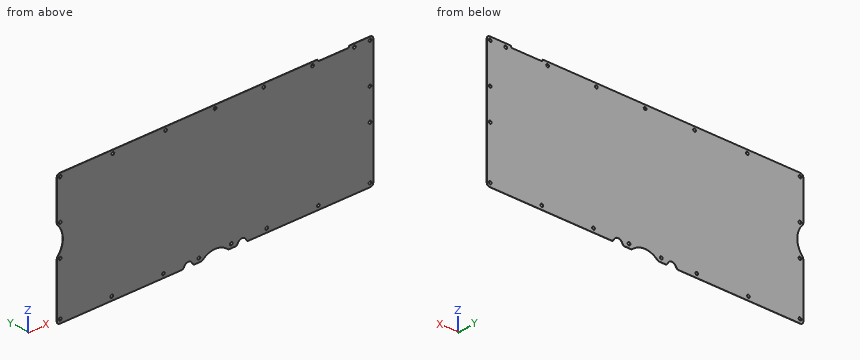
from build123d import *

# Parameters (mm, degrees)
SKETCH1_W                 = 373.38
SKETCH1_H                 = 149.225
BOSS_EXTRUDE1_DEPTH       = 0.254
F_4_CLEARANCE_HOLE2_D     = 3.2639
F_4_CLEARANCE_HOLE2_DEPTH = 0.762
F_4_CLEARANCE_HOLE2_TIP   = 0.980574487
CUT_EXTRUDE2_REACH        = 203.048
SKETCH7_R                 = 22.225
FILLET2_R                 = 3.175
F_4_CLEARANCE_HOLE3_D     = 3.2639
SKETCH10_R                = 5.334
CUT_EXTRUDE3_DEPTH        = 1.016
FILLET3_R                 = 3.175
SKETCH11_R                = 22.86
CUT_EXTRUDE4_DEPTH        = 202.047869355
FILLET4_R                 = 3.175
F_4_CLEARANCE_HOLE4_D     = 3.2639
SKETCH15_W                = 36.703
SKETCH15_H                = 2.6035
CUT_EXTRUDE5_DEPTH        = 202.047869355
F_4_CLEARANCE_HOLE5_D     = 3.2639
SKETCH20_W                = 373.38
SKETCH20_H                = 0.635
CUT_EXTRUDE6_DEPTH        = 202.047869355
FILLET6_R                 = 0.762
FILLET7_R                 = 3.175


with BuildPart() as part:
    # Sketch1 → Boss-Extrude1 (new body)
    with BuildSketch(Plane(origin=(0, 0, 0), x_dir=(1, 0, 0), z_dir=(0, 1, 0))):
        Rectangle(SKETCH1_W, SKETCH1_H)
    extrude(amount=BOSS_EXTRUDE1_DEPTH)

    # #4 Clearance Hole2
    with Locations(Plane(origin=(0, 0.254, 0), x_dir=(-1, 0, 0), z_dir=(0, 1, 0))):
        with Locations((121.92, -70.1675), (60.96, -70.1675), (0, -70.1675), (-60.96, -70.1675), (-121.92, -70.1675)):
            Hole(F_4_CLEARANCE_HOLE2_D / 2, depth=F_4_CLEARANCE_HOLE2_DEPTH)
            with Locations((0, 0, -(F_4_CLEARANCE_HOLE2_DEPTH + F_4_CLEARANCE_HOLE2_TIP / 2))):  # 118° drill point
                Cone(0, F_4_CLEARANCE_HOLE2_D / 2, F_4_CLEARANCE_HOLE2_TIP, mode=Mode.SUBTRACT)

    # Sketch7 → Cut-Extrude2 (cut, up to next)
    with BuildSketch(Plane(origin=(0, 0.254, 0), x_dir=(1, 0, 0), z_dir=(0, 1, 0)), mode=Mode.PRIVATE) as cut_extrude2_sk1:
        with Locations((0, 90.4875)):
            Circle(SKETCH7_R)
    cut_extrude2_tool1 = extrude(cut_extrude2_sk1.sketch, amount=-CUT_EXTRUDE2_REACH, mode=Mode.PRIVATE) & part.part
    add(cut_extrude2_tool1.solids().sort_by_distance((0, 0.254, -90.4875))[0], mode=Mode.SUBTRACT)

    # Fillet2
    fillet2_edges = [part.edges().sort_by_distance(p)[0] for p in [
        (15.554259867, 0.127, -74.6125),
        (-15.554259867, 0.127, -74.6125),
    ]]
    fillet(fillet2_edges, radius=FILLET2_R)

    # #4 Clearance Hole3 (through all)
    with Locations(Plane(origin=(0, 0.254, 0), x_dir=(-1, 0, 0), z_dir=(0, 1, 0))):
        with Locations((19.05, -70.1675), (-19.05, -70.1675)):
            Hole(F_4_CLEARANCE_HOLE3_D / 2)

    # Sketch10 → Cut-Extrude3 (cut)
    with BuildSketch(Plane(origin=(0, 0.254, 0), x_dir=(1, 0, 0), z_dir=(0, 1, 0))):
        with Locations((31.75, 74.6125)):
            Circle(SKETCH10_R)
        with Locations((-31.75, 74.6125)):
            Circle(SKETCH10_R)
    extrude(amount=-CUT_EXTRUDE3_DEPTH, mode=Mode.SUBTRACT)

    # Fillet3
    fillet3_edges = [part.edges().sort_by_distance(p)[0] for p in [
        (37.084, 0.127, -74.6125),
        (26.416, 0.127, -74.6125),
        (-26.416, 0.127, -74.6125),
        (-37.084, 0.127, -74.6125),
    ]]
    fillet(fillet3_edges, radius=FILLET3_R)

    # Sketch11 → Cut-Extrude4 (cut, through all)
    with BuildSketch(Plane(origin=(0, 0.254, 0), x_dir=(1, 0, 0), z_dir=(0, 1, 0))):
        with Locations((-202.565, -7.9375)):
            Circle(SKETCH11_R)
    extrude(amount=-CUT_EXTRUDE4_DEPTH, mode=Mode.SUBTRACT)

    # Fillet4
    fillet4_edges = [part.edges().sort_by_distance(p)[0] for p in [
        (-186.69, 0.127, -8.511328986),
        (-186.69, 0.127, 24.386328986),
        (-186.69, 0.127, -74.6125),
        (186.69, 0.127, -74.6125),
    ]]
    fillet(fillet4_edges, radius=FILLET4_R)

    # #4 Clearance Hole4 (through all)
    with Locations(Plane(origin=(0, 0.254, 0), x_dir=(-1, 0, 0), z_dir=(0, 1, 0))):
        with Locations((182.88, -70.1675), (182.88, -10.4775), (182.88, 25.0825), (182.88, 70.1675)):
            f_4_clearance_hole4 = Hole(F_4_CLEARANCE_HOLE4_D / 2)

    # Mirror1: #4 Clearance Hole4 across plane
    add(f_4_clearance_hole4.mirror(Plane(origin=(0, 0, 0), x_dir=(0, 0, 1), z_dir=(1, 0, 0))), mode=Mode.SUBTRACT)

    # Sketch15 → Cut-Extrude5 (cut, through all)
    with BuildSketch(Plane(origin=(0, 0.254, 0), x_dir=(1, 0, 0), z_dir=(0, 1, 0))):
        with Locations((139.7, -73.31075)):
            Rectangle(SKETCH15_W, SKETCH15_H)
    extrude(amount=-CUT_EXTRUDE5_DEPTH, mode=Mode.SUBTRACT)

    # #4 Clearance Hole5 (through all)
    with Locations(Plane(origin=(0, 0.254, 0), x_dir=(-1, 0, 0), z_dir=(0, 1, 0))):
        with Locations((-115.062, 70.1675), (-164.465, 70.1675), (0, 70.1675), (-57.531, 70.1675), (120.65, 70.1675), (58.42, 70.1675)):
            Hole(F_4_CLEARANCE_HOLE5_D / 2)

    # Sketch20 → Cut-Extrude6 (cut, through all)
    with BuildSketch(Plane(origin=(0, 0.254, 0), x_dir=(1, 0, 0), z_dir=(0, 1, 0))):
        with Locations((0, -74.295)):
            Rectangle(SKETCH20_W, SKETCH20_H)
    extrude(amount=-CUT_EXTRUDE6_DEPTH, mode=Mode.SUBTRACT)

    # Fillet6
    fillet6_edges = [part.edges().sort_by_distance(p)[0] for p in [
        (158.0515, 0.127, 72.009),
        (121.3485, 0.127, 72.009),
        (121.3485, 0.127, 73.9775),
        (158.0515, 0.127, 73.9775),
    ]]
    fillet(fillet6_edges, radius=FILLET6_R)

    # Fillet7
    fillet7_edges = [part.edges().sort_by_distance(p)[0] for p in [
        (-186.69, 0.127, 73.9775),
        (186.69, 0.127, 73.9775),
    ]]
    fillet(fillet7_edges, radius=FILLET7_R)


solid = part.part
Work out the finished part from the listing and answer in its coordinate system (mm). Give positions to 0.01 mm unless a question says otherwise; leave off trailing zeros. Loops run counter-clockwise (first coordinate to the right, second up) from the corner with the lowest first, then second, coordinate; pieces in that order, holes last. Notation, with made-up numbers: (74.25, 69) - (112.25, 69) arc R13 ccw to (112.25, 76) - close; hole circle Ø8 at (-25, 58). An arc over 180 degrees is marked (long way). Answer in a Markdown table with one row per item. Add a question column.
Q1. Consider line 1 along Z through (x, y) = (182.88, 0.1); line 2 along Z through (x, y) = (-182.88, 0.15); line 3 along Z through (x, y) = (-121.92, 0.2). Determine where each line is inside the solid, lowest interval first.
Q2. The part is cut by section A-A (z = 7.5). Determine the outline of the cut face in (x, y).
Q3. This flat-tipped pin is pushed along its axis until it touches: P1, Ø2, axis at x = 121.92, z = -70.17, coming from the +Y side. Where does it stop, or does it pass through?
Solution:
| question | item | result |
|---|---|---|
| 1 | line 1 | z = -74.61 to -71.8, -68.54 to -12.11, -8.85 to 23.45, 26.71 to 68.54, 71.8 to 73.98 |
| 1 | line 2 | z = -74.61 to -71.8, -68.54 to -12.11, -8.85 to -3.68, 19.56 to 23.45, 26.71 to 68.54, 71.8 to 73.98 |
| 1 | line 3 | z = -74.61 to -71.8, -68.54 to 69.14, 71.19 to 73.98 |
| 2 | outline | (-179.71, 0) - (186.69, 0) - (186.69, 0.25) - (-179.71, 0.25) - close |
| 3 | P1 | passes through |
